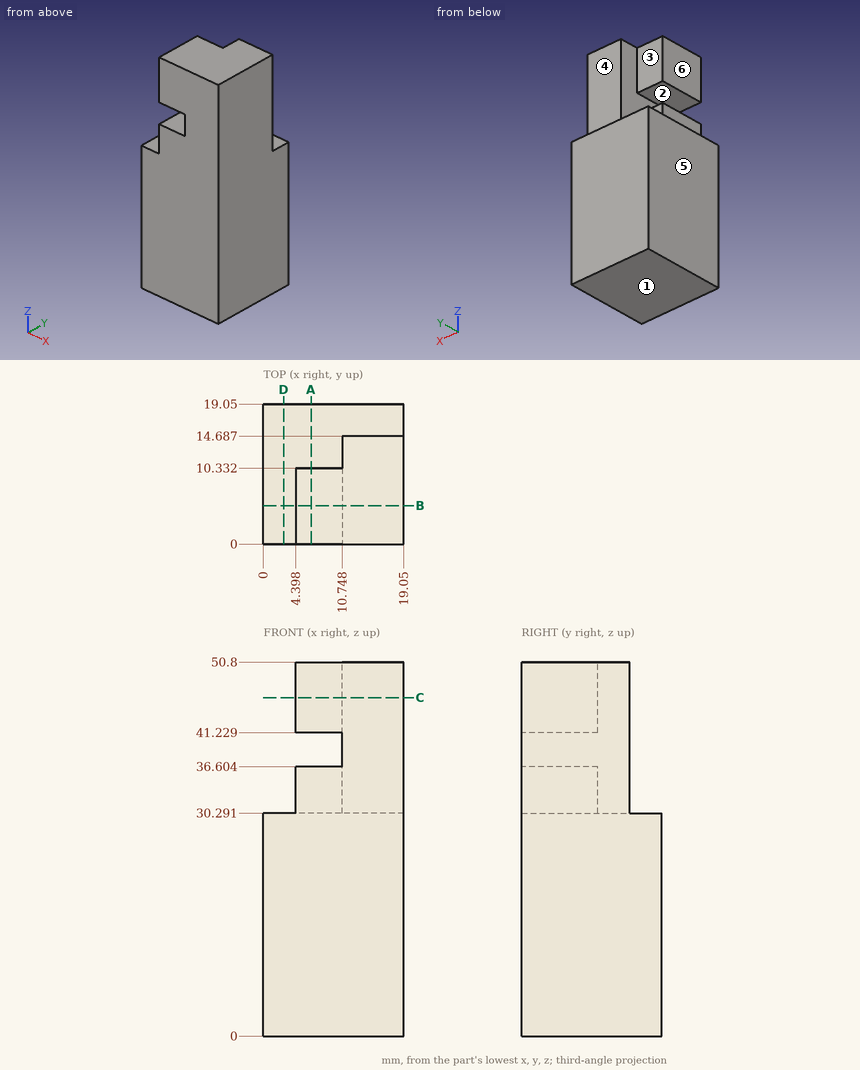
Input: dimensioned drawing with shaded views. Units: mm. Origin: part minimum x, y, z. A direction names the side the tool comes from. Coordinates: 2 decimals unless noted, no trailing zeros. Order: outer loops, then holes, each group sorted by start corner. A loop starts at its lowest first (then second) coordinate and runs counter-clockwise, first axis right, second up. Notation, with made-up numbers: (14.5, -13.5) - (51.5, -13.5) arc R20 ccw to (51.5, 9.5) - close; hole circle Ø4 at (73, 79). An arc over 180 degrees is marked (long way). Put each result on its own line as item: value.
1. Draft query along Z for the marked faces 1, 2 and 3. Return one class per face: pulls with the +Z half, pulls with the -Z half, needs draft (parallel to the pull), parting line crosses it, or undercut.
Report:
face 1: pulls with the -Z half
face 2: undercut
face 3: needs draft
2. Cut plane B-B on y = 5.25. Return the cut outline in (x, z), then the cut area to 3 significant figures.
Report:
outline: (0, 0) - (19.05, 0) - (19.05, 50.8) - (4.4, 50.8) - (4.4, 41.23) - (10.75, 41.23) - (10.75, 36.6) - (4.4, 36.6) - (4.4, 30.29) - (0, 30.29) - close
area: 848 mm2
3. Contact query for flat-ended pins moving along their axis: pin 1 Ø4 at (x, z) = (15.5, 43) entering from +Y; pin 2 Ø1.9 at (y, z) = (3.5, 32.5) entering from -X; pin 3 Ø7 at (x, z) = (6.5, 47) entering from +Y. Output: stop coordinate, or through.
Report:
pin 1: stops at y = 14.69
pin 2: stops at x = 4.4
pin 3: stops at y = 10.33
4. Cut plane A-A on x = 6.5. Return the cut outline in (y, z).
Report:
outline: (0, 0) - (19.05, 0) - (19.05, 30.29) - (10.33, 30.29) - (10.33, 36.6) - (0, 36.6) - close; (0, 41.23) - (10.33, 41.23) - (10.33, 50.8) - (0, 50.8) - close
5. Cut plane C-C on z = 46. Return the cut outline in (x, y).
Report:
outline: (4.4, 0) - (19.05, 0) - (19.05, 14.69) - (10.75, 14.69) - (10.75, 10.33) - (4.4, 10.33) - close
6. Line query: line 1 along Z through (x, y) = (7, 8); line 2 along Z through (x, y) = (3.75, 14); line 3 along Y through (x, z) = (13, 42.5). Output: solid intervals per line, ascending.
Report:
line 1: z = 0 to 36.6, 41.23 to 50.8
line 2: z = 0 to 30.29
line 3: y = 0 to 14.69
7. Cut plane D-D on x = 2.75. Return the cut outline in (y, z).
Report:
outline: (0, 0) - (19.05, 0) - (19.05, 30.29) - (0, 30.29) - close
8. Reachability of the marked faces 4, 5 and 6 from +Z, -Z, +X, -X, +Y, -Y: full face, straight path, thin tool, end or side. Return the list, or none.
Report:
face 4: +Z, +X, -X, +Y
face 5: +Z, -Z, -X, +Y, -Y
face 6: +Z, -X, +Y, -Y
